Autodesk Fusion 360 part; units mm, degrees
box "BoxPrimitive1" add length 139.7 width 292.1 height 19.05 placed x (0, 1, 0) y (-1, 0, 0) z (0, 0, 1) at (292.1, 0, 0)
fillet "Fillet1" radius 25.4 4 edges at (0, 0, 9.525) (0, 139.7, 9.525) (292.1, 0, 9.525) (292.1, 139.7, 9.525)
sketch "Sketch2" plane through (0, 0, 19.05) normal (0, 0, 1) x (-1, 0, 0)
  arc A0 (-292.1, -114.3) -> (-266.7, -139.7) centre (-266.7, -114.3) ccw
  line L0 (-266.7, -139.7) -> (-25.4, -139.7)
  arc A1 (-25.4, -139.7) -> (0, -114.3) centre (-25.4, -114.3) ccw
  line L1 (0, -114.3) -> (0, -25.4)
  arc A2 (0, -25.4) -> (-25.4, 0) centre (-25.4, -25.4) ccw
  line L2 (-25.4, 0) -> (-266.7, 0)
  arc A3 (-266.7, 0) -> (-292.1, -25.4) centre (-266.7, -25.4) ccw
  line L3 (-292.1, -25.4) -> (-292.1, -114.3)
  line L4 (-12.7, -114.3) -> (-12.7, -25.4)
  arc A4 (-12.7, -25.4) -> (-25.4, -12.7) centre (-25.4, -25.4) ccw
  line L5 (-25.4, -12.7) -> (-266.7, -12.7)
  arc A5 (-266.7, -12.7) -> (-279.4, -25.4) centre (-266.7, -25.4) ccw
  line L6 (-279.4, -25.4) -> (-279.4, -114.3)
  arc A6 (-279.4, -114.3) -> (-266.7, -127) centre (-266.7, -114.3) ccw
  line L7 (-266.7, -127) -> (-25.4, -127)
  arc A7 (-25.4, -127) -> (-12.7, -114.3) centre (-25.4, -114.3) ccw
  point P0 (-292.1, 0)
  point P1 (0, -139.7)
extrude "Extrude1" cut sketch "Sketch2" against normal blind 12.7 contours L4 A4 L5 A5 L6 A6 L7 A7
sketch "Sketch3" plane through (0, 0, 6.35) normal (0, 0, 1) x (-1, 0, 0)
  arc A0 (-25.4, -127) -> (-12.7, -114.3) centre (-25.4, -114.3) ccw
  line L0 (-12.7, -114.3) -> (-12.7, -25.4)
  arc A1 (-12.7, -25.4) -> (-25.4, -12.7) centre (-25.4, -25.4) ccw
  line L1 (-25.4, -12.7) -> (-266.7, -12.7)
  arc A2 (-266.7, -12.7) -> (-279.4, -25.4) centre (-266.7, -25.4) ccw
  line L2 (-279.4, -25.4) -> (-279.4, -114.3)
  arc A3 (-279.4, -114.3) -> (-266.7, -127) centre (-266.7, -114.3) ccw
  line L3 (-266.7, -127) -> (-25.4, -127)
  line L4 (-94.1365, -115.8394) -> (-131.1548, -115.8394)
  line L5 (-161.648, -99.7247) -> (-198.5274, -99.7247)
  line L6 (-161.6096, -40.1639) -> (-198.5361, -40.1639)
  line L7 (-93.4326, -23.8572) -> (-130.9835, -23.8572)
  line L8 (-93.4326, -23.8572) -> (-134.9646, -70.048)
  line L9 (-153.5362, -90.703) -> (-161.648, -99.7247)
  line L10 (-161.6096, -40.1639) -> (-153.5494, -49.2039)
  line L11 (-134.9646, -70.048) -> (-94.1365, -115.8394)
  line L12 (-130.9835, -23.8572) -> (-153.5494, -49.2039)
  line L13 (-172.017, -69.9473) -> (-198.5274, -99.7247)
  line L14 (-131.1548, -115.8394) -> (-153.5362, -90.703)
  line L15 (-172.017, -69.9473) -> (-198.5361, -40.1639)
extrude "Extrude2" add sketch "Sketch3" along normal blind 1.27 contours L4 L5 L6 L7 L8 L9 L10 L11 L12 L13 L14 L15
Design review of the part built by this model. Coordinates are the model's own, in mm. A direction names the side the tool comes from. Round coordinates to 2 decimals unless told otherwise and drop trailing zeros. Loops run counter-clockwise (first coordinate to the right, second up) from the corner with the lowest first, then second, coordinate; pieces in that order, holes last. Notation, with made-up numbers: (-3.5, -34) - (27.5, -34) arc R13 ccw to (27.5, -20) - close; hole circle Ø5 at (39, 37.5). An arc over 180 degrees is marked (long way). One line per item, written item: value. Start each with the question number.
1) For faces 1 (the flat face through (148, 139.7, 9)), 2 (the flat face through (113.91, 46.63, 6.98)), list the 3-axis set-ups (+Z, -Z, +X, -X, +Y, -Y) from which the entire face can be reached by the end or side of a thin tool; tool diameter is ignored.
2) Consider section B-B on x = 82. Give the boundary of the cut face in (y, z), then the cut area to 3 significant figures.
3) To check wall thickness, follow L1, parallel to X at y = 107.5, z = 11; L2, parallel to Y at x = 105, z = 9.5; L3, parallel to Y at x = 137, z = 6.5. State the ranges of each line that lie inside material, in increasing order. Write a range as from..to.
4) Draft analysis for pull direction X (two halves, no side actions). For faces 3 (the flat face through (147, 69, 7.62)), 4 (the flat face through (144, 69, 0)), 5 (the flat face through (292.1, 70, 9)), 6 (the cylindrical face through (7.64, 132.46, 9.66)), state which applies: +X half, -X half, draft (parallel to the pull), parting line (faces both ways), or undercut.
5) Consider section A-A on z = 11.25. Give the boundary of the cut face in (x, y).
6) Consider section D-D on y = 86. Give the boundary of the cut face in (x, z), then the cut area to 3 significant figures.
7) Insertion check: pin 1 Ø3 at (y, z) = (93.5, 3) entering from -X; pin 2 Ø1 at (x, y) = (122.5, 110) entering from +Z; pin 3 Ø1 at (x, y) = (87.5, 34.5) entering from +Z. Each pin has a flat end and moves straight along its axis. Give the tip position at first contact, or say it passes through.
8) Consider section C-C on y = 59.5. Give the boundary of the cut face in (x, z).
Reported:
1. face 1: +Z, -Z, +X, -X, +Y
1. face 2: +Z
2. outline: (0, 0) - (139.7, 0) - (139.7, 19.05) - (127, 19.05) - (127, 6.35) - (12.7, 6.35) - (12.7, 19.05) - (0, 19.05) - close
2. area: 1,210 mm^2
3. L1: x = 0..12.7, 279.4..292.1
3. L2: y = 0..12.7, 127..139.7
3. L3: y = 0..12.7, 30.62..109.27, 127..139.7
4. face 3: undercut
4. face 4: draft
4. face 5: +X half
4. face 6: -X half
5. outline: (0, 25.4) arc R25.4 ccw to (25.4, 0) - (266.7, 0) arc R25.4 ccw to (292.1, 25.4) - (292.1, 114.3) arc R25.4 ccw to (266.7, 139.7) - (25.4, 139.7) arc R25.4 ccw to (0, 114.3) - close; hole (12.7, 25.4) arc R12.7 ccw to (25.4, 12.7) - (266.7, 12.7) arc R12.7 ccw to (279.4, 25.4) - (279.4, 114.3) arc R12.7 ccw to (266.7, 127) - (25.4, 127) arc R12.7 ccw to (12.7, 114.3) - close
6. outline: (0, 0) - (292.1, 0) - (292.1, 19.05) - (279.4, 19.05) - (279.4, 6.35) - (186.31, 6.35) - (186.31, 7.62) - (120.74, 7.62) - (120.74, 6.35) - (12.7, 6.35) - (12.7, 19.05) - (0, 19.05) - close
6. area: 2,260 mm^2
7. pin 1: stops at x = 0
7. pin 2: stops at z = 7.62
7. pin 3: stops at z = 6.35
8. outline: (0, 0) - (292.1, 0) - (292.1, 19.05) - (279.4, 19.05) - (279.4, 6.35) - (181.32, 6.35) - (181.32, 7.62) - (125.48, 7.62) - (125.48, 6.35) - (12.7, 6.35) - (12.7, 19.05) - (0, 19.05) - close
